Check sheet for the modelled part. Datum: model origin and axes. Units: mm. A direction names the side the tool comes from. Coordinates: 2 decimals unless noted, no trailing zeros. Write each loop counter-clockwise with the first axis right and the second up, starting at its lowest first coordinate (ties: lowest second). Pieces come first, ordered by that corner, then holes. Notation, with made-up numbers: (9, 74) - (42, 74) arc R16 cw to (42, 92) - close; hole circle Ø11 at (-3, 41). An arc over 180 degrees is marked (long way). Use one line per item in the form item = value. Start each with the question number.
1. Draft check along X on faces 1 (the face through (17.03, 6.74, 2.96)), 2 (the face through (27.029, 7, 3)), 3 (the face through (-17.868, 2, 3)). Enter one of: +X half, -X half, draft (parallel to the pull), parting line (faces both ways), or undercut.
2. Cross-section at D-D on x = 3.5. Record the boundary of the cut face in (y, z).
3. Tool access check on faces 4 (the face through (23.95, 10.83, 2.96)), 5 (the face through (2, -0.582, 3)), 6 (the face through (23, 5.794, 3)), 7 (the face through (-1.55, -2.234, 2.958)). Record the directions out of +Z, -Z, +X, -X, +Y, -Y that give a thin tool (end or side, any length) a straight path to the whole face; none if there is none.
4. Cross-section at B-B on z = 3.5. Record the boundary of the cut face in (x, y), then the cut area to 3 significant figures.
5. Scan lines: line 1 along X through (y, z) = (2.25, 3.25); line 2 along Y through (x, z) = (5, 3); line 3 along X through (y, z) = (-1.75, 3). Record each from-to range of solid material in increasing order.
6. Go/stop test with flat-tipped pins: pin 1 Ø3 at (x, z) = (22, 3) entering from -Y; pin 2 Ø3 at (x, z) = (7, 4) entering from -Y; pin 3 Ø3.5 at (y, z) = (2, 4) entering from +X. Record where each tip stops, or that it passes through.
7. Cross-section at C-C on y = 6.25. Record the boundary of the cut face in (x, z).
8. Cross-section at A-A on x = -14.5. Record the boundary of the cut face in (y, z).
```python
from build123d import *

# Parameters (mm, degrees)
F1_DEPTH = 6
F2_SIZE  = 1.5


with BuildPart() as f1:
    # F0 (on Top) → F1 (new body)
    with BuildSketch(Plane.XY):
        Polygon((20.780653, 12.658395), (-1.74311, 12.658395), (-17.868141, 7.144866), (-17.868141, -2.784012), (-13.30795, -4.319267), (-3.109024, -10.286578), (0.33303, -10.286578), (2.583084, -0.582101), (1.663224, -0.582101), (0, -3.286578), (-3.143075, -1.150859), (-3.143075, 5.84374), (0, 7.658395), (15.440907, 7.658395), (18.67028, 5.793917), (27.028897, 5.793917), (27.028897, 9.05097), align=None)
        Polygon((-15.143075, 0.478634), (-15.143075, 3.478634), (-11.643075, 4.478634), (-8.143075, 3.478634), (-8.143075, 0.478634), (-11.643075, -0.521366), align=None, mode=Mode.SUBTRACT)
        Polygon((-13.30795, -4.319267), (-17.868141, -2.784012), (-17.868141, -3.318133), (-3.109024, -10.286578), align=None)
    extrude(amount=F1_DEPTH)

    # F2
    f2_edges = [f1.edges().sort_by_distance(p)[0] for p in [
        (9.518772, 12.658395, 6),
        (9.518772, 12.658395, 0),
    ]]
    chamfer(f2_edges, length=F2_SIZE)


solid = f1.part
```
Final values:
q1.face_1 = undercut
q1.face_2 = +X half
q1.face_3 = -X half
q2.outline = (7.66, 0) - (11.16, 0) - (12.66, 1.5) - (12.66, 4.5) - (11.16, 6) - (7.66, 6) - close
q3.face_4 = +Z, -Z, +X, +Y
q3.face_5 = +Z, -Z, +X
q3.face_6 = +Z, -Z, +X, -Y
q3.face_7 = +Z, -Z
q4.outline = (-17.87, -3.32) - (-3.11, -10.29) - (0.33, -10.29) - (2.58, -0.58) - (1.66, -0.58) - (0, -3.29) - (-3.14, -1.15) - (-3.14, 5.84) - (0, 7.66) - (15.44, 7.66) - (18.67, 5.79) - (27.03, 5.79) - (27.03, 9.05) - (20.78, 12.66) - (-1.74, 12.66) - (-17.87, 7.14) - close; hole (-15.14, 0.48) - (-11.64, -0.52) - (-8.14, 0.48) - (-8.14, 3.48) - (-11.64, 4.48) - (-15.14, 3.48) - close
q4.area = 412 mm²
q5.line_1 = -17.87 to -15.14, -8.14 to -3.14
q5.line_2 = 7.66 to 12.66
q5.line_3 = -17.87 to -2.26, 0.94 to 2.31
q6.pin_1 = 5.79
q6.pin_2 = 7.66
q6.pin_3 = -3.14
q7.outline = (-17.87, 0) - (-2.44, 0) - (-2.44, 6) - (-17.87, 6) - close; (17.88, 0) - (27.03, 0) - (27.03, 6) - (17.88, 6) - close
q8.outline = (-4.91, 0) - (0.29, 0) - (0.29, 6) - (-4.91, 6) - close; (3.66, 0) - (8.3, 0) - (8.3, 6) - (3.66, 6) - close
